Answer from the drawing. Dimensions are ordinates in mm from the lowest x, y and z of the part. Round coordinates to 2 decimals unless told otherwise and drop trailing zeros. Write each loop counter-clockwise with the first axis right and the second up, starting at its lowest first coordinate (ties: lowest second). Pieces come first, ordered by that corner, then holes.
1. Straight lines are drawn through the part: probe 1 along Y at (x, z) = (4, 4.4); probe 2 along X at (y, z) = (38, 7.25); probe 3 along Y at (x, z) = (6, 5.5). For each, find the intervals that lie inside material, in ascending order.
2. Find section D-D (y = 13). Write down the section's boundary in (x, z), and give its area (3 significant figures).
3. Flat-ended cylindrical pins translate along their axes: pin 1 Ø1.5 at (x, z) = (8.5, 5) entering from +Y; pin 2 Ø2 at (x, y) = (6, 13) entering from -Z; pin 3 Ø5 at (y, z) = (36, 4.4) entering from -X. Find the tip coordinate at first contact, or state that the pin passes through.
4. Find section C-C (x = 4.4). Write down the section's boundary in (y, z).
5. Find section B-B (y = 36). Write down the section's boundary in (x, z).
6. Find section A-A (z = 4.4). Write down the section's boundary in (x, y).
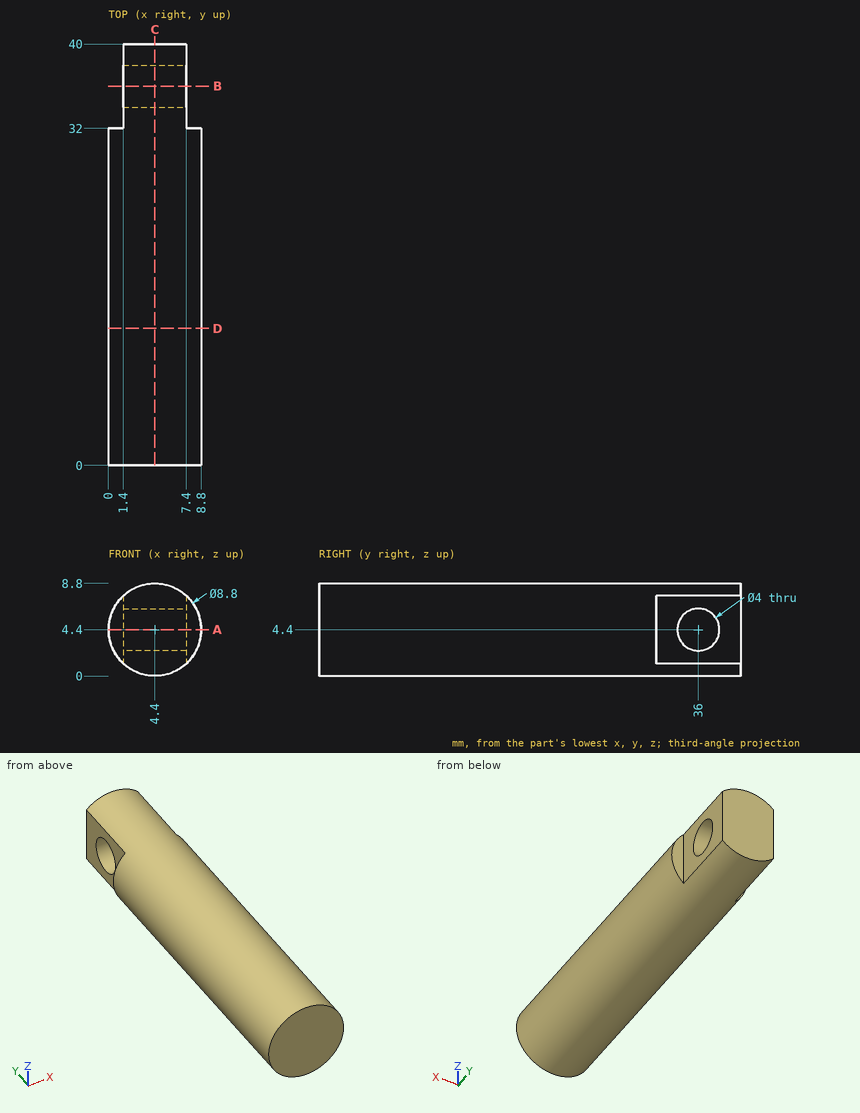
Worked answers:
1. probe 1: y = 0 to 34, 38 to 40
1. probe 2: x = 1.4 to 7.4
1. probe 3: y = 0 to 34.33, 37.67 to 40
2. outline: circle Ø8.8 at (4.4, 4.4)
2. area: 60.8 mm2
3. pin 1: stops at y = 32
3. pin 2: stops at z = 0.04
3. pin 3: stops at x = 1.4
4. outline: (0, 0) - (40, 0) - (40, 8.8) - (0, 8.8) - close; hole circle Ø4 at (36, 4.4)
5. outline: (1.4, 1.18) arc R4.4 ccw to (7.4, 1.18) - (7.4, 2.4) - (1.4, 2.4) - close; (1.4, 6.4) - (7.4, 6.4) - (7.4, 7.62) arc R4.4 ccw to (1.4, 7.62) - close
6. outline: (0, 0) - (8.8, 0) - (8.8, 32) - (7.4, 32) - (7.4, 34) - (1.4, 34) - (1.4, 32) - (0, 32) - close; (1.4, 38) - (7.4, 38) - (7.4, 40) - (1.4, 40) - close
